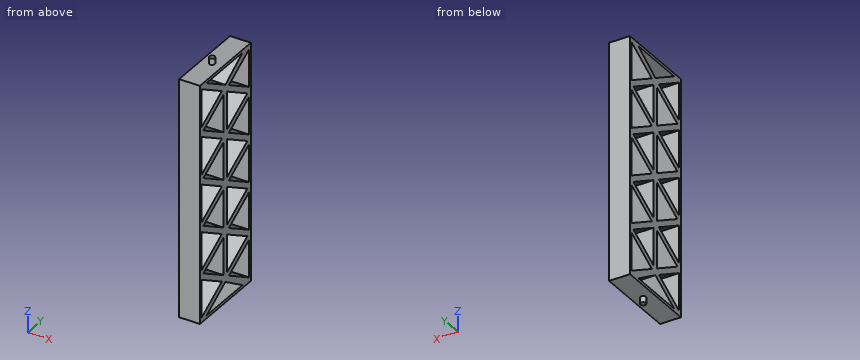
Autodesk Inventor part; units mm, degrees
ref_plane "YZ Plane" through (0, 0, 0) normal (1, 0, 0) x (0, 1, 0)
ref_plane "XZ Plane" through (0, 0, 0) normal (0, 1, 0) x (-1, 0, 0)
ref_plane "XY Plane" through (0, 0, 0) normal (0, 0, 1) x (1, 0, 0)
sketch "Sketch1" plane through (0, 0, 0) normal (1, 0, 0) x (0, 1, 0)
  line L0 (33.6396, 9.7397) -> (33.6396, -13.1356)
  line L1 (33.6396, -13.1356) -> (53.4502, -1.698)
  line L2 (53.4502, -1.698) -> (33.6396, 9.7397)
  line L3 (50.707, -1.698) -> (35.0112, -10.7599)
  line L4 (35.0112, -10.7599) -> (35.0112, 7.364)
  line L5 (35.0112, 7.364) -> (50.707, -1.698)
  line L6 (53.4502, -1.698) -> (33.6396, -13.1356)
  line L7 (53.4502, -24.5732) -> (33.6396, -13.1356)
  line L8 (53.4502, -1.698) -> (53.4502, -24.5732)
  line L9 (52.0786, -4.0736) -> (36.3828, -13.1356)
  line L10 (36.3828, -13.1356) -> (52.0786, -22.1975)
  line L11 (52.0786, -22.1975) -> (52.0786, -4.0736)
  line L12 (33.6396, -13.1356) -> (33.6396, -36.0108)
  line L13 (33.6396, -36.0108) -> (53.4502, -24.5732)
  line L14 (35.0112, -33.6351) -> (35.0112, -15.5113)
  line L15 (35.0112, -15.5113) -> (50.707, -24.5732)
  line L16 (50.707, -24.5732) -> (35.0112, -33.6351)
  line L17 (53.4502, -24.5732) -> (53.4502, -47.4484)
  line L18 (53.4502, -47.4484) -> (33.6396, -36.0108)
  line L19 (52.0786, -45.0728) -> (52.0786, -26.9489)
  line L20 (36.3828, -36.0108) -> (52.0786, -45.0728)
  line L21 (52.0786, -26.9489) -> (36.3828, -36.0108)
  line L22 (33.6396, -36.0108) -> (33.6396, -58.8861)
  line L23 (35.0112, -56.5104) -> (35.0112, -38.3865)
  line L24 (33.6396, -58.8861) -> (53.4502, -47.4484)
  line L25 (50.707, -47.4484) -> (35.0112, -56.5104)
  line L26 (35.0112, -38.3865) -> (50.707, -47.4484)
  line L27 (53.4502, -47.4484) -> (53.4502, -70.3237)
  line L28 (52.0786, -49.8241) -> (36.3828, -58.8861)
  line L29 (36.3828, -58.8861) -> (52.0786, -67.948)
  line L30 (53.4502, -70.3237) -> (33.6396, -58.8861)
  line L31 (52.0786, -67.948) -> (52.0786, -49.8241)
  line L32 (33.6396, -58.8861) -> (33.6396, -81.7613)
  line L33 (33.6396, -81.7613) -> (53.4502, -70.3237)
  line L34 (50.707, -70.3237) -> (35.0112, -79.3856)
  line L35 (35.0112, -79.3856) -> (35.0112, -61.2617)
  line L36 (35.0112, -61.2617) -> (50.707, -70.3237)
  line L37 (33.6396, -13.1356) -> (13.8291, -1.698)
  line L38 (13.8291, -1.698) -> (33.6396, 9.7397)
  line L39 (16.5723, -1.698) -> (32.268, -10.7599)
  line L40 (32.268, -10.7599) -> (32.268, 7.364)
  line L41 (32.268, 7.364) -> (16.5723, -1.698)
  line L42 (33.6396, -13.1356) -> (13.8291, -1.698)
  line L43 (13.8291, -24.5732) -> (33.6396, -13.1356)
  line L44 (13.8291, -1.698) -> (13.8291, -24.5732)
  line L45 (15.2007, -4.0736) -> (30.8964, -13.1356)
  line L46 (30.8964, -13.1356) -> (15.2007, -22.1975)
  line L47 (15.2007, -22.1975) -> (15.2007, -4.0736)
  line L48 (13.8291, -24.5732) -> (33.6396, -13.1356)
  line L49 (33.6396, -36.0108) -> (13.8291, -24.5732)
  line L50 (32.268, -15.5113) -> (16.5723, -24.5732)
  line L51 (32.268, -33.6351) -> (32.268, -15.5113)
  line L52 (16.5723, -24.5732) -> (32.268, -33.6351)
  line L53 (13.8291, -47.4484) -> (33.6396, -36.0108)
  line L54 (16.5723, -47.4484) -> (32.268, -56.5104)
  line L55 (32.268, -56.5104) -> (32.268, -38.3865)
  line L56 (33.6396, -58.8861) -> (13.8291, -47.4484)
  line L57 (32.268, -38.3865) -> (16.5723, -47.4484)
  line L58 (33.6396, -36.0108) -> (13.8291, -24.5732)
  line L59 (15.2007, -26.9489) -> (30.8964, -36.0108)
  line L60 (13.8291, -24.5732) -> (13.8291, -47.4484)
  line L61 (15.2007, -45.0728) -> (15.2007, -26.9489)
  line L62 (13.8291, -47.4484) -> (33.6396, -36.0108)
  line L63 (30.8964, -36.0108) -> (15.2007, -45.0728)
  line L64 (13.8291, -70.3237) -> (33.6396, -58.8861)
  line L65 (32.268, -79.3856) -> (32.268, -61.2617)
  line L66 (33.6396, -81.7613) -> (13.8291, -70.3237)
  line L67 (32.268, -61.2617) -> (16.5723, -70.3237)
  line L68 (16.5723, -70.3237) -> (32.268, -79.3856)
  line L69 (33.6396, -58.8861) -> (13.8291, -47.4484)
  line L70 (13.8291, -47.4484) -> (13.8291, -70.3237)
  line L71 (15.2007, -67.948) -> (15.2007, -49.8241)
  line L72 (15.2007, -49.8241) -> (30.8964, -58.8861)
  line L73 (13.8291, -70.3237) -> (33.6396, -58.8861)
  line L74 (30.8964, -58.8861) -> (15.2007, -67.948)
  line L75 (13.8291, -1.698) -> (13.8291, 21.1773)
  line L76 (13.8291, 21.1773) -> (33.6396, 9.7397)
  line L77 (53.4502, -1.698) -> (53.4502, 21.1773)
  line L78 (53.4502, 21.1773) -> (33.6396, 9.7397)
  line L79 (53.4502, 21.1773) -> (13.8291, 21.1773)
  line L80 (53.4502, -70.3237) -> (53.4502, -93.1989)
  line L81 (53.4502, -93.1989) -> (33.6396, -81.7613)
  line L82 (13.8291, -70.3237) -> (13.8291, -93.1989)
  line L83 (13.8291, -93.1989) -> (33.6396, -81.7613)
  line L84 (53.4502, -93.1989) -> (13.8291, -93.1989)
  line L85 (15.2007, 0.6777) -> (15.2007, 18.8016)
  line L86 (30.8964, 9.7397) -> (15.2007, 0.6777)
  line L87 (15.2007, 18.8016) -> (30.8964, 9.7397)
  line L88 (52.0786, 0.6777) -> (52.0786, 18.8016)
  line L89 (52.0786, 18.8016) -> (36.3828, 9.7397)
  line L90 (36.3828, 9.7397) -> (52.0786, 0.6777)
  line L91 (36.3828, -81.7613) -> (52.0786, -90.8232)
  line L92 (52.0786, -90.8232) -> (52.0786, -72.6994)
  line L93 (52.0786, -72.6994) -> (36.3828, -81.7613)
  line L94 (30.8964, -81.7613) -> (15.2007, -90.8232)
  line L95 (15.2007, -90.8232) -> (15.2007, -72.6994)
  line L96 (15.2007, -72.6994) -> (30.8964, -81.7613)
  line L97 (35.8485, 19.8048) -> (46.9126, 19.8048)
  line L98 (46.9126, 19.8048) -> (33.6396, 11.3245)
  line L99 (33.6396, 11.3245) -> (18.9514, 19.8048)
  line L100 (18.9514, 19.8048) -> (35.8485, 19.8048)
  line L101 (35.8485, -91.8264) -> (46.9126, -91.8264)
  line L102 (46.9126, -91.8264) -> (33.6396, -83.3461)
  line L103 (33.6396, -83.3461) -> (18.9514, -91.8264)
  line L104 (18.9514, -91.8264) -> (35.8485, -91.8264)
  dimension "d13" = 1.3716
extrude "Extrusion1" add sketch "Sketch1" along normal blind 10
sketch "Sketch2" plane through (0, 13.8291, 21.1773) normal (0, 0, 1) x (1, 0, 0)
  line L0 (0, 39.6211) -> (10, 39.6211)
  circle A0 centre (5.0038, 17.6108) radius 1.27
  point P0 (0, -13.8291)
  point P1 (0, 19.8105)
extrude "Extrusion2" add sketch "Sketch2" along normal blind 3
sketch "Sketch3" plane through (0, 13.8291, -93.1989) normal (0, 0, -1) x (-1, 0, 0)
  line L0 (0, 39.6211) -> (-10, 39.6211)
  line L1 (0, 21.1821) -> (-10, 21.1821)
  circle A0 centre (-5, 21.1821) radius 1.27
  point P0 (0, -13.8291)
  dimension "d36" = 2.54
extrude "Extrusion3" add sketch "Sketch3" along normal blind 3
properties part number "Arm support for middle arms"
CAD build for the part. Positions are in the model's coordinates, mm. Round coordinates to 2 decimals unless told otherwise and drop trailing zeros. Order: outer loops, then holes, each group sorted by start corner. A loop starts at its lowest first (then second) coordinate and runs counter-clockwise, first axis right, second up. Notation, with made-up numbers: (8.5, 38) - (39.5, 38) arc R24 ccw to (39.5, 76) - close; hole circle Ø11 at (80, 54). An arc over 180 degrees is marked (long way). Return JSON: item names as keys, results as strings.
(1) Cut at B-B (x = 5). State how many separate pieces and enclosed holes the cut face has, then the cut area to 3 significant figures.
Answer key:
{"separate pieces": "1", "enclosed holes": "20", "area": "1,750 mm^2"}
(2) Cut at D-D (z = -76.5). Give the cut face in (x, y), then the cut area to 3 significant figures.
Answer key:
{"outline": "(0, 13.83) - (10, 13.83) - (10, 15.2) - (0, 15.2) - close; (0, 21.78) - (10, 21.78) - (10, 27.27) - (0, 27.27) - close; (0, 32.27) - (10, 32.27) - (10, 35.01) - (0, 35.01) - close; (0, 40.01) - (10, 40.01) - (10, 45.5) - (0, 45.5) - close; (0, 52.08) - (10, 52.08) - (10, 53.45) - (0, 53.45) - close", "area": "165 mm^2"}
(3) Wall check: probe 1 along Y at (x, z) = (2, -38); probe 2 along Y at (x, z) = (1.5, 4); probe 3 along Y at (x, z) = (4, -62). Give the ranges that are in metal, low to high. Write a range as from..to.
Answer key:
{"probe 1": "y = 13.83..15.2, 27.45..39.83, 52.08..53.45", "probe 2": "y = 13.83..15.2, 20.96..26.44, 32.27..35.01, 40.84..46.32, 52.08..53.45", "probe 3": "y = 13.83..15.2, 25.5..30.99, 32.27..35.01, 36.29..41.78, 52.08..53.45"}
(4) Cut at A-A (z = 4). Give the cut face in (x, y), then the cut area to 3 significant figures.
Answer key:
{"outline": "(0, 13.83) - (10, 13.83) - (10, 15.2) - (0, 15.2) - close; (0, 20.96) - (10, 20.96) - (10, 26.44) - (0, 26.44) - close; (0, 32.27) - (10, 32.27) - (10, 35.01) - (0, 35.01) - close; (0, 40.84) - (10, 40.84) - (10, 46.32) - (0, 46.32) - close; (0, 52.08) - (10, 52.08) - (10, 53.45) - (0, 53.45) - close", "area": "165 mm^2"}
